```python
from build123d import *

# Parameters (mm, degrees)
F0_R     = 5
F0_W     = 72
F0_H     = 23
F1_DEPTH = 2
F0_W_2   = 8
F0_H_2   = 2
F0_W_3   = 3
F2_DEPTH = 6.25
F3_R     = 3
F5_DEPTH = 2
F4_W     = 12
F4_H     = 2
F6_DEPTH = 15
F7_R     = 3


with BuildPart() as f1:
    # F0 (on Front) → F1 (new body)
    with BuildSketch(Plane.XZ):
        with BuildLine():
            Line((29.867854, 38.356669), (-52.132146, 38.356669))
            Line((-52.132146, 38.356669), (-52.132146, -27.643331))
            Line((-52.132146, -27.643331), (-44.132146, -27.643331))
            Line((-44.132146, -27.643331), (-44.132146, -25.393331))
            Line((-44.132146, -25.393331), (-24.132146, -25.393331))
            Line((-24.132146, -25.393331), (-24.132146, -27.643331))
            Line((-24.132146, -27.643331), (-21.132146, -27.643331))
            Line((-21.132146, -27.643331), (-21.132146, -25.393331))
            Line((-21.132146, -25.393331), (-1.132146, -25.393331))
            Line((-1.132146, -25.393331), (-1.132146, -27.643331))
            Line((-1.132146, -27.643331), (6.867854, -27.643331))
            Line((6.867854, -27.643331), (6.867854, -1.643331))
            Line((6.867854, -1.643331), (26.867854, -1.643331))
            ThreePointArc((26.867854, -1.643331), (28.989174, -0.764651), (29.867854, 1.356669))
            Line((29.867854, 1.356669), (29.867854, 38.356669))
        make_face()
        with Locations((-34.132146, -14.643331)):
            Circle(F0_R, mode=Mode.SUBTRACT)
        with Locations((-11.132146, -14.643331)):
            Circle(F0_R, mode=Mode.SUBTRACT)
        with Locations((-11.132146, 14.856669)):
            Rectangle(F0_W, F0_H, mode=Mode.SUBTRACT)
    extrude(amount=F1_DEPTH)

    # F0 (on Front) → F2 (join)
    with BuildSketch(Plane.XZ):
        with Locations((-48.132146, -28.643331)):
            Rectangle(F0_W_2, F0_H_2)
        with Locations((-22.632146, -28.643331)):
            Rectangle(F0_W_3, F0_H_2)
        with Locations((2.867854, -28.643331)):
            Rectangle(F0_W_2, F0_H_2)
    extrude(amount=F2_DEPTH)

    # F3
    f3_edges = [f1.edges().sort_by_distance(p)[0] for p in [
        (-48.132146, 0, -29.643331),
        (-22.632146, 0, -29.643331),
        (2.867854, 0, -29.643331),
    ]]
    fillet(f3_edges, radius=F3_R)

    # F4 (on face) → F5 (join)
    with BuildSketch(Plane.XY.offset(38.356669)):
        Polygon((-52.132146, 8), (-52.132146, 0), (29.867854, 0), (29.867854, 8), (-5.132146, 49), (-5.132146, 77), (-17.132146, 77), (-17.132146, 49), align=None)
    extrude(amount=-F5_DEPTH)

    # F4 (on face) → F6 (join)
    with BuildSketch(Plane.XY.offset(38.356669)):
        with Locations((-11.132146, 78)):
            Rectangle(F4_W, F4_H)
    extrude(amount=-F6_DEPTH)

    # F7
    f7_edges = [f1.edges().sort_by_distance(p)[0] for p in [
        (-11.132146, 79, 38.356669),
        (-11.132146, -2, 38.356669),
    ]]
    fillet(f7_edges, radius=F7_R)


solid = f1.part
```
Check sheet for the modelled part. Datum: model origin and axes. Units: mm. A direction names the side the tool comes from. Round coordinates to 2 decimals unless told otherwise and drop trailing zeros. Write each loop counter-clockwise with the first axis right and the second up, starting at its lowest first coordinate (ties: lowest second). Pieces come first, ordered by that corner, then holes. Notation, with made-up numbers: M 60,14.5 L 81,14.5 A30 cw 81,51.5 Z; hole C -35,-10 d1. An arc over 180 degrees is marked long. Write item = value, one per line. Start each with the question number.
1. Section check C-C, the plane x = -14. Record the cut outline in (y, z).
2. Section check B-B, the plane x = 15. Record the cut outline in (y, z).
3. Tool access check on faces 1 (the flat face through (-11, 77, 30)), 2 (the flat face through (-5.132, 67, 37)), 3 (the flat face through (-48, -4, -27.643)), 4 (the flat face through (-24.132, -3, -28)). Record the directions out of +Z, -Z, +X, -X, +Y, -Y that give a thin tool (end or side, any length) a straight path to the whole face; none if there is none.
4. Section check D-D, the plane z = 27.5. Record the cut outline in (x, y).
5. Scan lines: line 1 (Y direction, x = -10.5, z = -5); line 2 (Z direction, x = 10.5, y = 15). Record each from-to range of solid material in increasing order. Write a range as [from, to].
6. Section check A-A, the plane z = 8.5. Record the cut outline in (x, y), then the cut area to 3 significant figures.
7. Gauge pin test, flat ends, axial feed: pin 1 (1.3 mm diameter, centred on x = -49.5, y = -3.5, fed in from +Z); pin 2 (8 mm diameter, centred on x = -11.13, z = -14.64, fed in from -Y); pin 3 (3.5 mm diameter, centred on x = -10.5, z = 32, fed in from -Y); pin 4 (12 mm diameter, centred on x = 1, z = -20, fed in from +Y). Record the tip position at first contact, or that the pin passes through.
8. Release check for a two-part mould opening along Z. For faces 5 (the flat face through (-21.132, -3, -28)), 6 (the cylindrical face through (-15.1, -0.986, -17.686)), 7 (the cylindrical face through (-22.611, -0.855, -28.741)) record: pulls with the +Z half, pulls with the -Z half, needs draft (parallel to the pull), parting line crosses it, or undercut.
Results found:
q1.outline = M -2,-25.39 L 0,-25.39 L 0,-18.74 L -2,-18.74 Z; M -2,-10.55 L 0,-10.55 L 0,3.36 L -2,3.36 Z; M -2,26.36 L 0,26.36 L 0,36.36 L 77,36.36 L 77,23.36 L 79,23.36 L 79,35.36 A3 ccw 76,38.36 L 1,38.36 A3 ccw -2,35.36 Z
q2.outline = M -2,-1.64 L 0,-1.64 L 0,3.36 L -2,3.36 Z; M -2,26.36 L 0,26.36 L 0,36.36 L 25.42,36.36 L 25.42,38.36 L 1,38.36 A3 ccw -2,35.36 Z
q3.face_1 = -Z, +X, -X
q3.face_2 = +Z, -Z, +X, +Y
q3.face_3 = +Z, +X, -X, -Y
q3.face_4 = -Z, +Y, -Y
q4.outline = M -52.13,-2 L 29.87,-2 L 29.87,0 L -52.13,0 Z; M -17.13,77 L -5.13,77 L -5.13,79 L -17.13,79 Z
q5.line_1 = [-2, 0]
q5.line_2 = [36.36, 38.36]
q6.outline = M -52.13,-2 L -47.13,-2 L -47.13,0 L -52.13,0 Z; M 24.87,-2 L 29.87,-2 L 29.87,0 L 24.87,0 Z
q6.area = 20.0 mm^2
q7.pin_1 = -27.64
q7.pin_2 = through
q7.pin_3 = -2
q7.pin_4 = 0
q8.face_5 = needs draft
q8.face_6 = undercut
q8.face_7 = pulls with the -Z half
